Job drawing, mm, ordinate dimensions from the low corner. One solid piece. Round coordinates to 2 decimals unless told otherwise and drop trailing zeros. Loops run counter-clockwise (first coordinate to the right, second up) from the corner with the lowest first, then second, coordinate; pieces in that order, holes last. Notation, with made-up numbers: M 36.25,43 L 42.25,43 A31 ccw 42.25,73 Z; hole C 66,41 d10. An arc over 180 degrees is marked long. Use a Markdown table: item, result. Add a question column.
(1) Wall check: L1, parallel to X at y = 0.5, z = 13; L2, parallel to Z at x = 6, y = 1. Give the ranges that are in metal, low to high.
(2) Band-saw the part on B-B, the plane y = 3.25. Give the number of separate pieces and of enclosed holes in the cut face, and give its area (3 significant figures).
(3) Band-saw the part on C-C, the plane x = 15. Write the cut outline in (y, z), and give its area (3 significant figures).
(4) Band-saw the part on A-A, the plane z = 105. Write the cut outline in (x, y), and give its area (3 significant figures).
(5) Flat gauge pin, fed straight in: P1, Ø3, axis at x = 123.5, z = 44.5, coming from the +Y side. Where does the tip first touch, or does it go through?
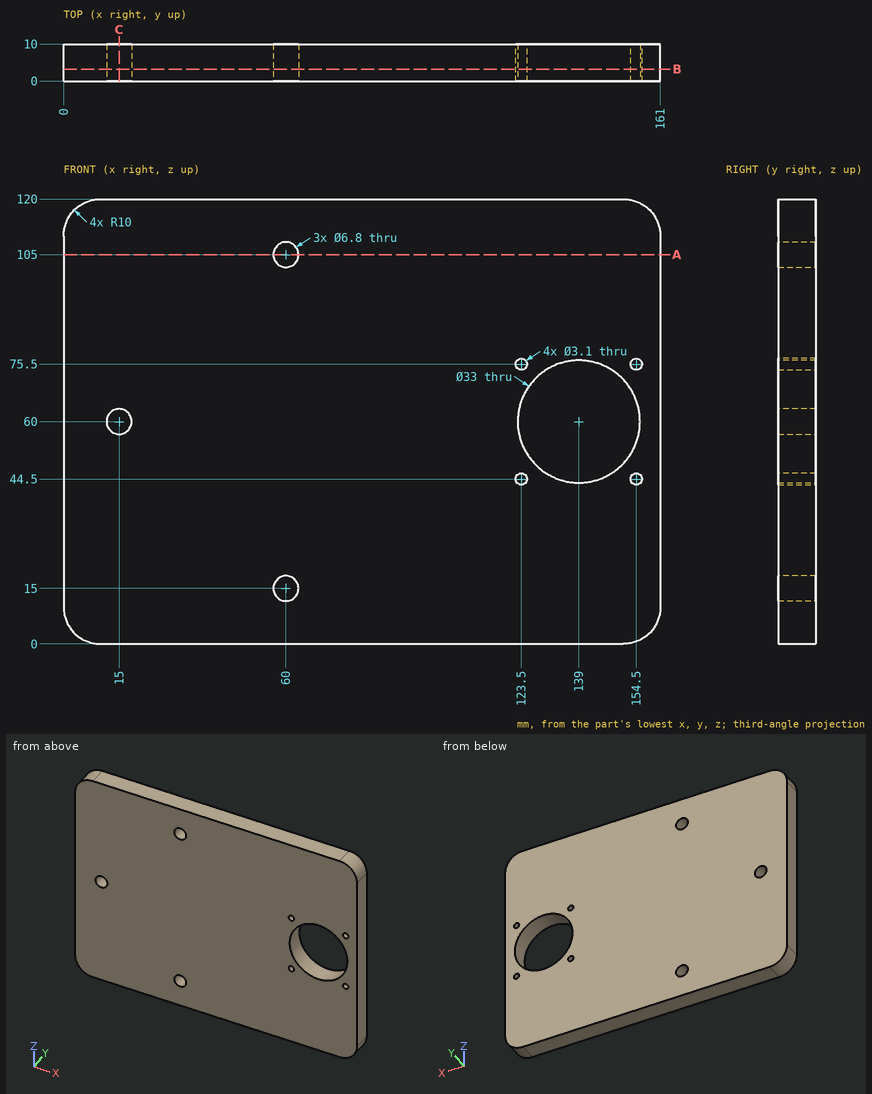
Return value:
| question | item | result |
|---|---|---|
| 1 | L1 | 0 to 57.25, 62.75 to 161 |
| 1 | L2 | 0.83 to 119.17 |
| 2 | separate pieces | 1 |
| 2 | enclosed holes | 8 |
| 2 | area | 18,200 mm^2 |
| 3 | outline | M 0,0 L 10,0 L 10,56.6 L 0,56.6 Z; M 0,63.4 L 10,63.4 L 10,120 L 0,120 Z |
| 3 | area | 1,130 mm^2 |
| 4 | outline | M 0,0 L 56.6,0 L 56.6,10 L 0,10 Z; M 63.4,0 L 161,0 L 161,10 L 63.4,10 Z |
| 4 | area | 1,540 mm^2 |
| 5 | P1 | through |
